Can you work these out from the model? Positions are in its coordinate system, mm. A direction names the side the tool comes from. Coordinates: 2 decimals unless noted, no trailing zeros. Loops run counter-clockwise (first coordinate to the right, second up) from the corner with the lowest first, then second, coordinate; pieces in that order, holes last. Notation, with made-up numbers: (7, -2) -> (60, -2) arc R14 ccw to (60, 9) -> close; hole circle Ø2 at (61, 25). An arc over 180 degrees is marked (long way). Use one line per item in the form item = value. Start each with the question number.
(1) On a 3-axis mill with a long thin cutter (end or side, diameter ignored), from which of +Z, -Z, +X, -X, +Y, -Y can I reach the whole of each face in a straight line? I mean faces 4 (the flat face through (30, 20, -12)), 5 (the flat face through (-9.3, 0.3, 15)), 6 (the flat face through (30, 11, -16.5)). Say none if no direction works.
(2) Imagine slicing it at C-C (y = 14.25). List the corners of the cut face in (x, z) for me, plus the area to 3 significant figures.
(3) I'm going to push flat-ended pins straight in: pin 1 (2 mm diameter, centred on x = -30, z = 0, fed in from +Y); pin 2 (1.1 mm diameter, centred on x = 31, y = 20.5, fed in from +Z); pin 3 (6 mm diameter, centred on x = 23, z = 10.5, fed in from -Y); pin 4 (8 mm diameter, centred on x = -22, y = 7.5, fed in from -Z). Where does each tip first touch, or does it pass through?
(4) I need wall thicknesses on line 1 (Z direction, x = 31.5, y = 4); line 2 (X direction, y = 0.5, z = 0); line 3 (X direction, y = 19, z = 2). Which ranges of each line are inside material? Lowest first, please. Write a range as [from, to].
(5) Thinking about a two-plate mould opening in Y: for faces 1 (the flat face through (1, 0, 0)), 2 (the flat face through (25, 13, 17)), 3 (the flat face through (-28, 20, 0)), which applies, released by +Y, released by -Y, zero draft, split by the parting line, or undercut?
(6) Imagine slicing it at B-B (z = -14). List the corners of the cut face in (x, y) for me.
(7) Imagine slicing it at D-D (x = -30). List the corners of the cut face in (y, z) for me.
(8) Imagine slicing it at A-A (x = -20). List the corners of the cut face in (y, z) for me, plus the area to 3 significant figures.
```python
from build123d import *

# Parameters (mm, degrees)
T_LE_DE_BASE_PLI_E1_DEPTH               = 1
T_LE_PLI_E_SUR_AR_TE1_STRIP_W           = 5.4732
T_LE_PLI_E_SUR_AR_TE1_STRIP_H           = 1
T_LE_PLI_E_SUR_AR_TE1_STRIP_CUT_DEPTH   = 30
T_LE_PLI_E_SUR_AR_TE1_DEPTH             = 30
T_LE_PLI_E_SUR_AR_TE2_STRIP_W           = 5.4732
T_LE_PLI_E_SUR_AR_TE2_STRIP_H           = 1
T_LE_PLI_E_SUR_AR_TE2_STRIP_CUT_DEPTH   = 30
T_LE_PLI_E_SUR_AR_TE2_DEPTH             = 30
ENL_V_MAT_EXTRU_1_REACH                 = 46.026
ESQUISSE12_R                            = 1.7
ENL_V_MAT_EXTRU_3_REACH                 = 45.557
ESQUISSE27_R                            = 2.25
T_LE_PLI_E_SUR_AR_TE3_STRIP_W           = 5.4732
T_LE_PLI_E_SUR_AR_TE3_STRIP_H           = 1
T_LE_PLI_E_SUR_AR_TE3_STRIP_CUT_DEPTH   = 10
T_LE_PLI_E_SUR_AR_TE3_STRIP_2_W         = 5.4732
T_LE_PLI_E_SUR_AR_TE3_STRIP_2_H         = 1
T_LE_PLI_E_SUR_AR_TE3_STRIP_CUT_2_DEPTH = 10
T_LE_PLI_E_SUR_AR_TE3_DEPTH             = 10
T_LE_PLI_E_SUR_AR_TE3_BEND_DEPTH        = 10
T_LE_PLI_E_SUR_AR_TE4_STRIP_W           = 5.4732
T_LE_PLI_E_SUR_AR_TE4_STRIP_H           = 1
T_LE_PLI_E_SUR_AR_TE4_STRIP_CUT_DEPTH   = 10
T_LE_PLI_E_SUR_AR_TE4_STRIP_2_W         = 5.4732
T_LE_PLI_E_SUR_AR_TE4_STRIP_2_H         = 1
T_LE_PLI_E_SUR_AR_TE4_STRIP_CUT_2_DEPTH = 10
T_LE_PLI_E_SUR_AR_TE4_DEPTH             = 10
T_LE_PLI_E_SUR_AR_TE4_BEND_DEPTH        = 10
ENL_V_MAT_EXTRU_2_REACH                 = 46.41
ESQUISSE26_R                            = 1.7


# Sheet-metal steps are written as plain solids
with BuildPart() as part:
    # Esquisse1 → Tôle de base pliée1 (new body)
    with BuildSketch(Plane(origin=(0, 0, 0), x_dir=(1, 0, 0), z_dir=(0, 1, 0))):
        Polygon((35, -15), (35, -16.5), (25, -16.5), (25, -15), (-35, -15), (-35, 15), (25, 15), (25, 16.5), (35, 16.5), (35, 15), align=None)
    extrude(amount=T_LE_DE_BASE_PLI_E1_DEPTH)

    # Tôle pliée sur arête1 strip (across the edge) → Tôle pliée sur arête1 strip cut (cut)
    with BuildSketch(Plane(origin=(-35, 1, -15), x_dir=(1, 0, 0), z_dir=(0, 0, 1))):
        with Locations((-1, -0.5)):
            Rectangle(T_LE_PLI_E_SUR_AR_TE1_STRIP_W, T_LE_PLI_E_SUR_AR_TE1_STRIP_H)
    extrude(amount=T_LE_PLI_E_SUR_AR_TE1_STRIP_CUT_DEPTH, mode=Mode.SUBTRACT)

    # Tôle pliée sur arête1 section (across the edge) → Tôle pliée sur arête1 (add)
    with BuildSketch(Plane(origin=(-35, 1, -15), x_dir=(1, 0, 0), z_dir=(0, 0, 1))):
        with BuildLine():
            Line((0, 0.7366), (0, 20))
            Line((0, 20), (1, 20))
            Line((1, 20), (1, 0.7366))
            ThreePointArc((1, 0.7366), (1.215745145, 0.215745145), (1.7366, 0))
            Line((1.7366, 0), (1.7366, -1))
            ThreePointArc((1.7366, -1), (0.508638364, -0.491361636), (0, 0.7366))
        make_face()
    extrude(amount=T_LE_PLI_E_SUR_AR_TE1_DEPTH)

    # Tôle pliée sur arête2 strip (across the edge) → Tôle pliée sur arête2 strip cut (cut)
    with BuildSketch(Plane(origin=(-34, 21, -15), x_dir=(0, -1, 0), z_dir=(0, 0, 1))):
        with Locations((-1, -0.5)):
            Rectangle(T_LE_PLI_E_SUR_AR_TE2_STRIP_W, T_LE_PLI_E_SUR_AR_TE2_STRIP_H)
    extrude(amount=T_LE_PLI_E_SUR_AR_TE2_STRIP_CUT_DEPTH, mode=Mode.SUBTRACT)

    # Tôle pliée sur arête2 section (across the edge) → Tôle pliée sur arête2 (add)
    with BuildSketch(Plane(origin=(-34, 21, -15), x_dir=(0, -1, 0), z_dir=(0, 0, 1))):
        with BuildLine():
            Line((0, 0.7366), (0, 7))
            Line((0, 7), (1, 7))
            Line((1, 7), (1, 0.7366))
            ThreePointArc((1, 0.7366), (1.215745145, 0.215745145), (1.7366, 0))
            Line((1.7366, 0), (1.7366, -1))
            ThreePointArc((1.7366, -1), (0.508638364, -0.491361636), (0, 0.7366))
        make_face()
    extrude(amount=T_LE_PLI_E_SUR_AR_TE2_DEPTH)

    # Esquisse12 → Enlèv. mat.-Extru.1 (cut, up to next)
    with BuildSketch(Plane(origin=(0, 21, 0), x_dir=(1, 0, 0), z_dir=(0, 1, 0)), mode=Mode.PRIVATE) as enl_v_mat_extru_1_sk1:
        with Locations(Location((-30, 0, 0), (0, 0, 180))):
            Circle(ESQUISSE12_R)
    enl_v_mat_extru_1_tool1 = extrude(enl_v_mat_extru_1_sk1.sketch, amount=-ENL_V_MAT_EXTRU_1_REACH, mode=Mode.PRIVATE) & part.part
    add(enl_v_mat_extru_1_tool1.solids().sort_by_distance((-30, 21, 0))[0], mode=Mode.SUBTRACT)

    # Esquisse27 → Enlèv. mat.-Extru.3 (cut, up to next)
    with BuildSketch(Plane(origin=(0, 1, 0), x_dir=(1, 0, 0), z_dir=(0, 1, 0)), mode=Mode.PRIVATE) as enl_v_mat_extru_3_sk1:
        with Locations(Location((-20, 0, 0), (0, 0, 270))):
            Circle(ESQUISSE27_R)
    enl_v_mat_extru_3_tool1 = extrude(enl_v_mat_extru_3_sk1.sketch, amount=-ENL_V_MAT_EXTRU_3_REACH, mode=Mode.PRIVATE) & part.part
    # Esquisse27 → Enlèv. mat.-Extru.3 (cut, up to next)
    with BuildSketch(Plane(origin=(0, 1, 0), x_dir=(1, 0, 0), z_dir=(0, 1, 0)), mode=Mode.PRIVATE) as enl_v_mat_extru_3_sk2:
        with Locations(Location((20, 0, 0), (0, 0, 270))):
            Circle(ESQUISSE27_R)
    enl_v_mat_extru_3_tool2 = extrude(enl_v_mat_extru_3_sk2.sketch, amount=-ENL_V_MAT_EXTRU_3_REACH, mode=Mode.PRIVATE) & part.part
    add(enl_v_mat_extru_3_tool1.solids().sort_by_distance((-20, 1, 0))[0], mode=Mode.SUBTRACT)
    add(enl_v_mat_extru_3_tool2.solids().sort_by_distance((20, 1, 0))[0], mode=Mode.SUBTRACT)

    # Tôle pliée sur arête3 strip (across the edge) → Tôle pliée sur arête3 strip cut (cut)
    with BuildSketch(Plane(origin=(25, 1, 16.5), x_dir=(0, 0, -1), z_dir=(1, 0, 0))):
        with Locations((-2, -0.5)):
            Rectangle(T_LE_PLI_E_SUR_AR_TE3_STRIP_W, T_LE_PLI_E_SUR_AR_TE3_STRIP_H)
    extrude(amount=T_LE_PLI_E_SUR_AR_TE3_STRIP_CUT_DEPTH, mode=Mode.SUBTRACT)

    # Tôle pliée sur arête3 strip 2 (across the edge) → Tôle pliée sur arête3 strip cut 2 (cut)
    with BuildSketch(Plane(origin=(35, 1, -16.5), x_dir=(0, 0, 1), z_dir=(-1, 0, 0))):
        with Locations((-2, -0.5)):
            Rectangle(T_LE_PLI_E_SUR_AR_TE3_STRIP_2_W, T_LE_PLI_E_SUR_AR_TE3_STRIP_2_H)
    extrude(amount=T_LE_PLI_E_SUR_AR_TE3_STRIP_CUT_2_DEPTH, mode=Mode.SUBTRACT)

    # Tôle pliée sur arête3 section (across the edge) → Tôle pliée sur arête3 (add)
    with BuildSketch(Plane(origin=(25, 1, 16.5), x_dir=(0, 0, -1), z_dir=(1, 0, 0))):
        with BuildLine():
            Line((-1, 0.7366), (-1, 19))
            Line((-1, 19), (0, 19))
            Line((0, 19), (0, 0.7366))
            ThreePointArc((0, 0.7366), (0.215745145, 0.215745145), (0.7366, 0))
            Line((0.7366, 0), (0.7366, -1))
            ThreePointArc((0.7366, -1), (-0.491361636, -0.491361636), (-1, 0.7366))
        make_face()
    extrude(amount=T_LE_PLI_E_SUR_AR_TE3_DEPTH)

    # Tôle pliée sur arête3 section 2 (across the edge) → Tôle pliée sur arête3 bend (add)
    with BuildSketch(Plane(origin=(35, 1, -16.5), x_dir=(0, 0, 1), z_dir=(-1, 0, 0))):
        with BuildLine():
            Line((-1, 0.7366), (-1, 19))
            Line((-1, 19), (0, 19))
            Line((0, 19), (0, 0.7366))
            ThreePointArc((0, 0.7366), (0.215745145, 0.215745145), (0.7366, 0))
            Line((0.7366, 0), (0.7366, -1))
            ThreePointArc((0.7366, -1), (-0.491361636, -0.491361636), (-1, 0.7366))
        make_face()
    extrude(amount=T_LE_PLI_E_SUR_AR_TE3_BEND_DEPTH)

    # Tôle pliée sur arête4 strip (across the edge) → Tôle pliée sur arête4 strip cut (cut)
    with BuildSketch(Plane(origin=(25, 20, 16.5), x_dir=(0, -1, 0), z_dir=(1, 0, 0))):
        with Locations((-2, -0.5)):
            Rectangle(T_LE_PLI_E_SUR_AR_TE4_STRIP_W, T_LE_PLI_E_SUR_AR_TE4_STRIP_H)
    extrude(amount=T_LE_PLI_E_SUR_AR_TE4_STRIP_CUT_DEPTH, mode=Mode.SUBTRACT)

    # Tôle pliée sur arête4 strip 2 (across the edge) → Tôle pliée sur arête4 strip cut 2 (cut)
    with BuildSketch(Plane(origin=(35, 20, -16.5), x_dir=(0, -1, 0), z_dir=(-1, 0, 0))):
        with Locations((-2, -0.5)):
            Rectangle(T_LE_PLI_E_SUR_AR_TE4_STRIP_2_W, T_LE_PLI_E_SUR_AR_TE4_STRIP_2_H)
    extrude(amount=T_LE_PLI_E_SUR_AR_TE4_STRIP_CUT_2_DEPTH, mode=Mode.SUBTRACT)

    # Tôle pliée sur arête4 section (across the edge) → Tôle pliée sur arête4 (add)
    with BuildSketch(Plane(origin=(25, 20, 16.5), x_dir=(0, -1, 0), z_dir=(1, 0, 0))):
        with BuildLine():
            Line((-1, 0.7366), (-1, 11))
            Line((-1, 11), (0, 11))
            Line((0, 11), (0, 0.7366))
            ThreePointArc((0, 0.7366), (0.215745145, 0.215745145), (0.7366, 0))
            Line((0.7366, 0), (0.7366, -1))
            ThreePointArc((0.7366, -1), (-0.491361636, -0.491361636), (-1, 0.7366))
        make_face()
    extrude(amount=T_LE_PLI_E_SUR_AR_TE4_DEPTH)

    # Tôle pliée sur arête4 section 2 (across the edge) → Tôle pliée sur arête4 bend (add)
    with BuildSketch(Plane(origin=(35, 20, -16.5), x_dir=(0, -1, 0), z_dir=(-1, 0, 0))):
        with BuildLine():
            Line((-1, 0.7366), (-1, 11))
            Line((-1, 11), (0, 11))
            Line((0, 11), (0, 0.7366))
            ThreePointArc((0, 0.7366), (0.215745145, 0.215745145), (0.7366, 0))
            Line((0.7366, 0), (0.7366, -1))
            ThreePointArc((0.7366, -1), (-0.491361636, -0.491361636), (-1, 0.7366))
        make_face()
    extrude(amount=T_LE_PLI_E_SUR_AR_TE4_BEND_DEPTH)

    # Esquisse26 → Enlèv. mat.-Extru.2 (cut, up to next)
    with BuildSketch(Plane(origin=(0, 21, 0), x_dir=(1, 0, 0), z_dir=(0, 1, 0)), mode=Mode.PRIVATE) as enl_v_mat_extru_2_sk1:
        with Locations(Location((30, -10, 0), (0, 0, 270))):
            Circle(ESQUISSE26_R)
    enl_v_mat_extru_2_tool1 = extrude(enl_v_mat_extru_2_sk1.sketch, amount=-ENL_V_MAT_EXTRU_2_REACH, mode=Mode.PRIVATE) & part.part
    # Esquisse26 → Enlèv. mat.-Extru.2 (cut, up to next)
    with BuildSketch(Plane(origin=(0, 21, 0), x_dir=(1, 0, 0), z_dir=(0, 1, 0)), mode=Mode.PRIVATE) as enl_v_mat_extru_2_sk2:
        with Locations(Location((30, 10, 0), (0, 0, 90))):
            Circle(ESQUISSE26_R)
    enl_v_mat_extru_2_tool2 = extrude(enl_v_mat_extru_2_sk2.sketch, amount=-ENL_V_MAT_EXTRU_2_REACH, mode=Mode.PRIVATE) & part.part
    add(enl_v_mat_extru_2_tool1.solids().sort_by_distance((30, 21, 10))[0], mode=Mode.SUBTRACT)
    add(enl_v_mat_extru_2_tool2.solids().sort_by_distance((30, 21, -10))[0], mode=Mode.SUBTRACT)


solid = part.part
```
Worked out:
q1.face_4 = +X
q1.face_5 = +Z, -X, +Y, -Y
q1.face_6 = +X, -X
q2.outline = (-35, -15) -> (-34, -15) -> (-34, 15) -> (-35, 15) -> close; (25, -17.5) -> (35, -17.5) -> (35, -16.5) -> (25, -16.5) -> close; (25, 16.5) -> (35, 16.5) -> (35, 17.5) -> (25, 17.5) -> close
q2.area = 50.0 mm2
q3.pin_1 = 1
q3.pin_2 = 17.36
q3.pin_3 = 0
q3.pin_4 = through
q4.line_1 = [-17.5, -16.5], [16.5, 17.5]
q4.line_2 = [-34.48, -22.25], [-17.75, 17.75], [22.25, 35]
q4.line_3 = [-35, -34]
q5.face_1 = released by -Y
q5.face_2 = zero draft
q5.face_3 = undercut
q6.outline = (-35, 1.74) arc R1.74 ccw to (-33.26, 0) -> (35, 0) -> (35, 1) -> (-33.26, 1) arc R0.74 cw to (-34, 1.74) -> (-34, 19.26) arc R0.74 cw to (-33.26, 20) -> (-27, 20) -> (-27, 21) -> (-33.26, 21) arc R1.74 ccw to (-35, 19.26) -> close; (25, 20) -> (35, 20) -> (35, 21) -> (25, 21) -> close
q7.outline = (0, -15) -> (1, -15) -> (1, 15) -> (0, 15) -> close; (20, -15) -> (21, -15) -> (21, -1.7) -> (20, -1.7) -> close; (20, 1.7) -> (21, 1.7) -> (21, 15) -> (20, 15) -> close
q8.outline = (0, -15) -> (1, -15) -> (1, -2.25) -> (0, -2.25) -> close; (0, 2.25) -> (1, 2.25) -> (1, 15) -> (0, 15) -> close
q8.area = 25.5 mm2
